Input: part model. Units: mm. Frame: model coordinates. A direction names the side the tool comes from. Round coordinates to 2 decimals unless told otherwise and drop trailing zeros. Loops run counter-clockwise (first coordinate to the right, second up) from the corner with the lowest first, then second, coordinate; pieces in that order, holes last. Notation, with made-up numbers: (64.5, 21) -> (76.5, 21) arc R24 ccw to (76.5, 39) -> close; hole circle Ø8 at (28, 0). An arc over 180 degrees is marked (long way). One line per question, with ' | ' between items. Start each with the question number.
Q1. Cut plane A-A on y = 0. State how many separate pieces and enclosed holes the cut face has, and give its area (3 significant figures).
Q2. Material intervals for L1, parallel to Y at x = 4, z = -1; L2, parallel to Z at x = 10.25, y = -4; L3, parallel to Y at x = 7.5, z = 0, sorted ascending.
Q3. Cut plane D-D on x = 3.5. Return loops of the section in (y, z).
Q4. Contact query for flat-ended pins moving along their axis: P1, Ø1.2, axis at x = 15, z = 1.5, coming from the -Y side; P2, Ø1.2, axis at x = 15.5, y = -0.5, coming from the -Z side; P3, Ø4.5, axis at x = 15, z = 1.5, coming from the +Y side. Output: stop coordinate, or through.
Q5. Cut plane B-B on x = 13.75. Return loops of the section in (y, z).
Q6. Mould query, pull axis Z, two halves, no side actions, for faces 6 (the face through (15, 0, -4.1)), 7 (the face through (13, -2, 2)), 8 (the face through (3.472, -15.368, -2.018)), 9 (the face through (1.5, -4, 10)). Classes: pulls with the +Z half, pulls with the -Z half, needs draft (parallel to the pull), parting line crosses it, or undercut.
Q7. Access query for faces 1 (the face through (15, -4.1, 0)), 2 (the face through (7, 1, 2.2)), 3 (the face through (3.528, -0.336, 11.494)), 4 (the face through (7.69, -10.007, -0.04)), 5 (the face through (7.69, 10.007, 0.04)). Directions: +Z, -Z, +X, -X, +Y, -Y. A direction counts if a zero-diameter tool reaches every point of the face in a straight line with its end or side. Return the directions, or none.
from build123d import *

# Parameters (mm, degrees)
ESQUISSE2_R                  = 9.539549542
ESQUISSE2_W                  = 8.2
ESQUISSE2_H                  = 8.2
BOSS_EXTRU_1_DEPTH           = 4
ESQUISSE3_R                  = 1.55
ENL_V_MAT_EXTRU_1_DEPTH      = 25.753787589
ESQUISSE4_R                  = 3
ENL_V_MAT_EXTRU_2_DEPTH      = 25.753787589
R_P_TITION_CIRCULAIRE1_COUNT = 4


with BuildPart() as part:
    # Esquisse1 → Révolution1 (revolve)
    with BuildSketch(Plane.XY, mode=Mode.PRIVATE) as r_volution1_sk:
        Polygon((1.5, 15.5), (1.5, 10.514205948), (11, 8), (11, 5), (7, 5), (7, 2.1), (13, 2.1), (13, 9.539549542), (5.5, 11.524448975), (5.5, 15.5), align=None)
    revolve(r_volution1_sk.sketch.rotate(Axis((0, 0, 0), (1, 0, 0)), 90), axis=Axis((0, 0, 0), (1, 0, 0)))

    # Esquisse2 → Boss.-Extru.1 (add)
    with BuildSketch(Plane(origin=(13, 0, 0), x_dir=(0, 0, -1), z_dir=(1, 0, 0))):
        Circle(ESQUISSE2_R)
        Rectangle(ESQUISSE2_W, ESQUISSE2_H, mode=Mode.SUBTRACT)
    extrude(amount=BOSS_EXTRU_1_DEPTH)

    # Esquisse3 → Enlèv. mat.-Extru.1 (cut, through all)
    with BuildSketch(Plane(origin=(5.5, 0, 0), x_dir=(0, 0, -1), z_dir=(1, 0, 0))):
        with Locations((0, 13.007102974)):
            Circle(ESQUISSE3_R)
    enl_v_mat_extru_1 = extrude(amount=-ENL_V_MAT_EXTRU_1_DEPTH, mode=Mode.SUBTRACT)

    # Esquisse4 → Enlèv. mat.-Extru.2 (cut, through all)
    with BuildSketch(Plane(origin=(5.5, 0, 0), x_dir=(0, 0, -1), z_dir=(1, 0, 0))):
        with Locations((0, 13.007102974)):
            Circle(ESQUISSE4_R)
    enl_v_mat_extru_2 = extrude(amount=ENL_V_MAT_EXTRU_2_DEPTH, mode=Mode.SUBTRACT)

    # Répétition circulaire1: Enlèv. mat.-Extru.1, Enlèv. mat.-Extru.2 ×4 about axis
    r_p_tition_circulaire1_axis = Axis((0, 0, 0), (1, 0, 0))
    add([enl_v_mat_extru_1.rotate(r_p_tition_circulaire1_axis, i * 360 / R_P_TITION_CIRCULAIRE1_COUNT) for i in range(1, R_P_TITION_CIRCULAIRE1_COUNT)], mode=Mode.SUBTRACT)
    add([enl_v_mat_extru_2.rotate(r_p_tition_circulaire1_axis, i * 360 / R_P_TITION_CIRCULAIRE1_COUNT) for i in range(1, R_P_TITION_CIRCULAIRE1_COUNT)], mode=Mode.SUBTRACT)


solid = part.part
Results:
1) separate pieces: 4 | enclosed holes: 0 | area: 131 mm^2
2) L1: -15.47 to -14.19, -11.82 to -9.8, 9.8 to 11.82, 14.19 to 15.47 | L2: -9.46 to -7.16, -3 to 3, 7.16 to 9.46 | L3: -10.01 to -8.93, -5 to -2.1, 2.1 to 5, 8.93 to 10.01
3) outline: circle Ø31 at (0, 0); hole circle Ø3.1 at (-13.01, 0); hole circle Ø19.97 at (0, 0); hole circle Ø3.1 at (0, -13.01); hole circle Ø3.1 at (0, 13.01); hole circle Ø3.1 at (13.01, 0)
4) P1: y = -9.5 | P2: z = -9.54 | P3: y = 9.54
5) outline: circle Ø19.08 at (0, 0); hole (-4.1, -4.1) -> (4.1, -4.1) -> (4.1, 4.1) -> (-4.1, 4.1) -> close
6) face 6: undercut | face 7: undercut | face 8: parting line crosses it | face 9: needs draft
7) face 1: +X | face 2: -X | face 3: +X, -X | face 4: +X, -Y | face 5: +X, +Y
